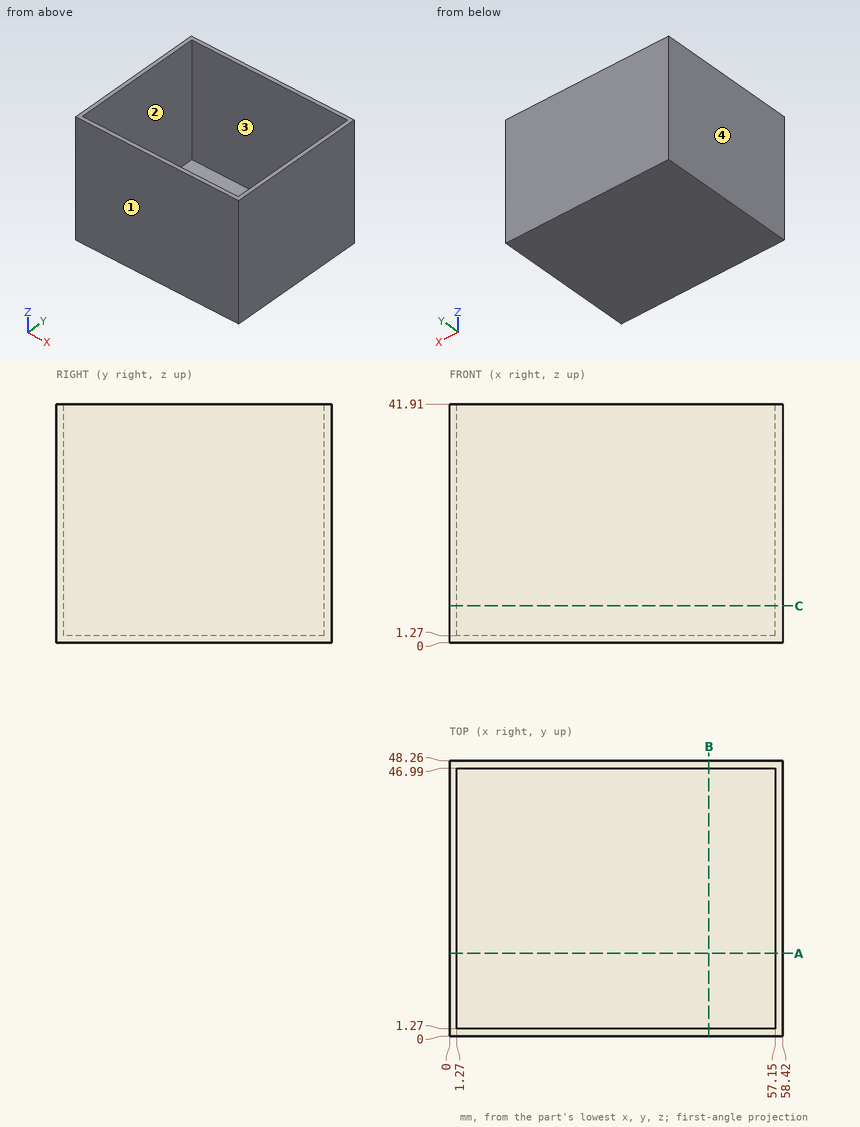
Here's the drawing with two shaded views (mm, measured from the low corner). I have some questions. Round coordinates to 2 decimals unless told otherwise and drop trailing zeros. Order: outer loops, then holes, each group sorted by start corner. A loop starts at its lowest first (then second) coordinate and runs counter-clockwise, first axis right, second up. Notation, with made-up numbers: (43.25, -2) -> (57.25, -2) arc R15 cw to (57.25, 22) -> close; hole circle Ø4 at (28, 73.25). An arc over 180 degrees is marked (long way). Use a Markdown table: item, result. Add a question column.
(1) Suppose I cut it at C-C, the plane z = 6.5. Please give me the cut outline in (x, y).
(2) If we mould it in two halves opening along Y, with no side actions, what happens to the marked faces 1, 2, 3 and 4? For each: released by +Y, released by -Y, zero draft, split by the parting line, or undercut.
(3) Suppose I cut it at A-A, the plane y = 14.5. Please give me the cut outline in (x, z), and give its area (3 significant figures).
(4) Suppose I cut it at B-B, the plane x = 45.5. Please give me the cut outline in (y, z).
(5) I need wall thicknesses on line 1 along Y through (x, z) = (39.5, 20.5); line 2 along X through (y, z) = (26, 18.5); line 3 along Z through (x, y) = (38, 35.5). Which ranges of each line are inside material? Lowest first, please.
(6) For pin 1 Ø23 at (x, y) = (31, 19) entering from +Z, with a flat end and sliding along its axis, tell me the tip position at first contact or that it passes through.
Verdict:
| question | item | result |
|---|---|---|
| 1 | outline | (0, 0) -> (58.42, 0) -> (58.42, 48.26) -> (0, 48.26) -> close; hole (1.27, 1.27) -> (57.15, 1.27) -> (57.15, 46.99) -> (1.27, 46.99) -> close |
| 2 | face 1 | released by -Y |
| 2 | face 2 | undercut |
| 2 | face 3 | undercut |
| 2 | face 4 | zero draft |
| 3 | outline | (0, 0) -> (58.42, 0) -> (58.42, 41.91) -> (57.15, 41.91) -> (57.15, 1.27) -> (1.27, 1.27) -> (1.27, 41.91) -> (0, 41.91) -> close |
| 3 | area | 177 mm2 |
| 4 | outline | (0, 0) -> (48.26, 0) -> (48.26, 41.91) -> (46.99, 41.91) -> (46.99, 1.27) -> (1.27, 1.27) -> (1.27, 41.91) -> (0, 41.91) -> close |
| 5 | line 1 | 0 to 1.27, 46.99 to 48.26 |
| 5 | line 2 | 0 to 1.27, 57.15 to 58.42 |
| 5 | line 3 | 0 to 1.27 |
| 6 | pin 1 | z = 1.27 |
